Autodesk Inventor part; units mm, degrees
ref_plane "YZ Plane" through (0, 0, 0) normal (1, 0, 0) x (0, 1, 0)
ref_plane "XZ Plane" through (0, 0, 0) normal (0, 1, 0) x (-1, 0, 0)
ref_plane "XY Plane" through (0, 0, 0) normal (0, 0, 1) x (1, 0, 0)
sketch "Sketch1" plane through (0, 0, 0) normal (0, 0, 1) x (1, 0, 0)
  line L0 (0, 0) -> (0, 75)
  line L1 (0, 0) -> (100, 0)
  line L2 (100, 0) -> (100, 75)
  line L3 (0, 75) -> (2, 75)
  line L4 (2, 75) -> (2, 2)
  line L5 (2, 2) -> (98, 2)
  line L6 (98, 2) -> (98, 75)
  line L7 (98, 75) -> (100, 75)
  dimension "d0" = 75
  dimension "d1" = 100
  dimension "d2" = 75
  dimension "d3" = 2
  dimension "d4" = 73
  dimension "d5" = 96
extrude "Extrusion1" add sketch "Sketch1" against normal blind 100
sketch "Sketch2" plane through (100, 0, 0) normal (1, 0, 0) x (0, 0, -1)
  line L0 (0, 75) -> (100, 75)
  line L1 (0, 75) -> (20, 75)
  line L2 (100, 2) -> (100, 75)
  line L3 (20, 75) -> (20, 62)
  line L4 (20, 62) -> (80, 62)
  circle A0 centre (20, 62) radius 7.5
  circle A1 centre (80, 62) radius 7.5
  point P0 (0, 0)
  dimension "d8" = 20
  dimension "d9" = 13
  dimension "d10" = 60
  dimension "d11" = 15
  dimension "d12" = 15
extrude "Extrusion2" cut sketch "Sketch2" against normal through all
properties part number "motor holder"
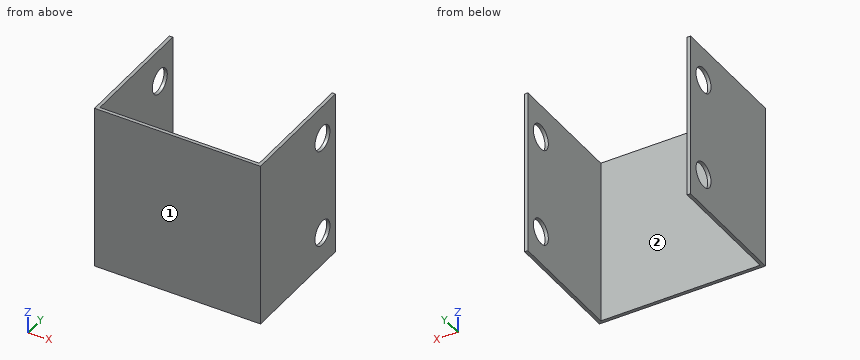
Could you check a few things on this model? Use its own coordinates, in mm. Face numbers are marked on the shaded views. A direction names the side the tool comes from. Give positions to 0.01 mm unless a question says otherwise; leave off trailing zeros. Order: outer loops, then holes, each group sorted by start corner. A loop starts at its lowest first (then second) coordinate and runs counter-clockwise, first axis right, second up. Notation, with made-up numbers: (67.25, 22) - (101.25, 22) arc R16 ccw to (101.25, 45) - close; hole circle Ø5 at (86.25, 31). An arc over 180 degrees is marked (long way). Return JSON: item names as keys, results as strings. Group by question number.
Q1. Suppose I cut it at B-B, the plane y = 62. Please give me the cut outline in (x, z), and give its area (3 significant figures).
Q2. Will this pin go through, and if not, where does the flat tip stop? pin 1 Ø3 at (x, z) = (35.5, -60) entering from +Y.
Q3. Please list where these lines run through material, in increasing order: line 1 along Z through (x, y) = (99, 62); line 2 along X through (y, z) = (5.5, -38.5); line 3 along Y through (x, z) = (1.65, -20). Write a range as [from, to].
Q4. Suppose I cut it at D-D, the plane z = -59. Please give me the cut outline in (x, y), and give its area (3 significant figures).
Q5. Which directions (+Z, -Z, +X, -X, +Y, -Y) give clear straight access to the entire face, cutting with the end or side of a thin tool? Please do the marked faces 1 and 2.
Q6. Suppose I cut it at A-A, the plane y = 16. Please give me the cut outline in (x, z).
Q7. Suppose I cut it at C-C, the plane z = -80. Please give me the cut outline in (x, y), and give its area (3 significant figures).
Resolved:
{
 "1": {"outline": "(0, -100) - (2, -100) - (2, -87.5) - (0, -87.5) - close; (0, -72.5) - (2, -72.5) - (2, -27.5) - (0, -27.5) - close; (0, -12.5) - (2, -12.5) - (2, 0) - (0, 0) - close; (98, -100) - (100, -100) - (100, -87.5) - (98, -87.5) - close; (98, -72.5) - (100, -72.5) - (100, -27.5) - (98, -27.5) - close; (98, -12.5) - (100, -12.5) - (100, 0) - (98, 0) - close", "area": "280 mm2"},
 "2": {"pin 1": "stops at y = 2"},
 "3": {"line 1": "z = [-100, -87.5], [-72.5, -27.5], [-12.5, 0]", "line 2": "x = [0, 2], [98, 100]", "line 3": "y = [0, 54.5], [69.5, 75]"},
 "4": {"outline": "(0, 0) - (100, 0) - (100, 75) - (98, 75) - (98, 2) - (2, 2) - (2, 75) - (0, 75) - close", "area": "492 mm2"},
 "5": {"face 1": "+Z, -Z, +X, -X, -Y", "face 2": "+Z, -Z, +Y"},
 "6": {"outline": "(0, -100) - (2, -100) - (2, 0) - (0, 0) - close; (98, -100) - (100, -100) - (100, 0) - (98, 0) - close"},
 "7": {"outline": "(0, 0) - (100, 0) - (100, 54.5) - (98, 54.5) - (98, 2) - (2, 2) - (2, 54.5) - (0, 54.5) - close; (0, 69.5) - (2, 69.5) - (2, 75) - (0, 75) - close; (98, 69.5) - (100, 69.5) - (100, 75) - (98, 75) - close", "area": "432 mm2"}
}
